Part print with two shaded views. Sizes in mm from the minimum x, y, z corner. A direction names the side the tool comes from. Give positions to 0.01 mm unless a question says otherwise; leave off trailing zeros. Write each loop counter-clockwise with the first axis right and the second up, starting at its lowest first coordinate (ties: lowest second). Pieces come first, ordered by that corner, then holes.
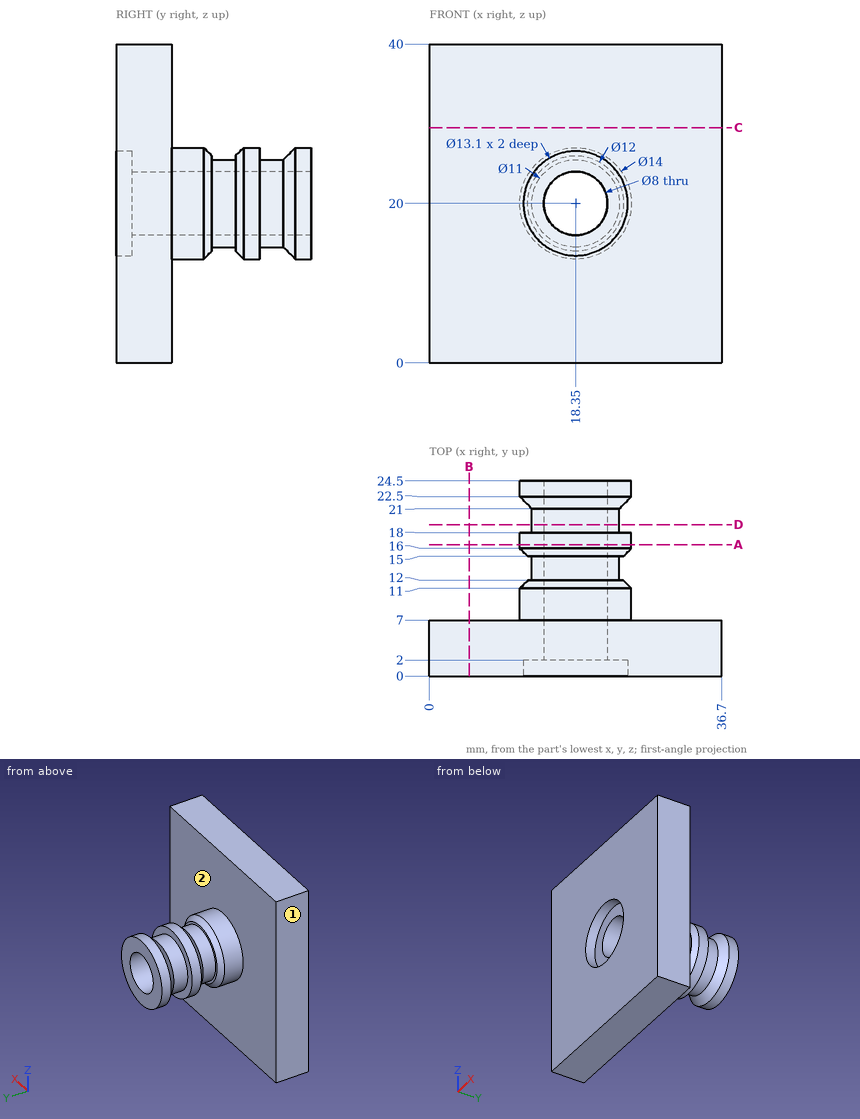
(1) Drop flat-ended pins along their axis: pin 1 (4 mm diameter, centred on x = 31.5, z = 32.5, fed in from +Y); pin 2 (8 mm diameter, centred on x = 12.5, y = 17, fed in from +Z). Give the stop position or say it passes through.
(2) 3-axis set-ups, long thin cutter, end or side, ignore diameter. For the marked faces 1 and 2: which of +Z, -Z, +X, -X, +Y, -Y reach the whole face in a straight line?
(3) Saw through at C-C, the plane z = 29.5. List the corners of the cut face in (x, y).
(4) Probe line 1 (X direction, y = 3.15, z = 20); line 2 (Z direction, x = 18.35, y = 17.5); line 3 (Y direction, x = 31.5, z = 22). List the from-to ranges inside material, lowest first.
(5) Saw through at D-D, the plane y = 19. List the corners of the cut face in (x, z).
(6) Saw through at B-B, the plane x = 5. List the corners of the cut face in (y, z), plus the area to 3 significant figures.
(7) Saw through at A-A, the plane y = 16.5. List the corners of the cut face in (x, z), plus the area to 3 significant figures.
Computed values:
1. pin 1: stops at y = 7
1. pin 2: stops at z = 26.75
2. face 1: +Z, -Z, -X, +Y, -Y
2. face 2: +Y
3. outline: (0, 0) - (36.7, 0) - (36.7, 7) - (0, 7) - close
4. line 1: x = 0 to 14.35, 22.35 to 36.7
4. line 2: z = 13 to 16, 24 to 27
4. line 3: y = 0 to 7
5. outline: circle Ø11 at (18.35, 20); hole circle Ø8 at (18.35, 20)
6. outline: (0, 0) - (7, 0) - (7, 40) - (0, 40) - close
6. area: 280 mm2
7. outline: circle Ø14 at (18.35, 20); hole circle Ø8 at (18.35, 20)
7. area: 104 mm2
